Solid Edge part; units mm, degrees
sketch "Sketch1" plane through (0, 0, 0) normal (1, 0, 0) x (0, 1, 0)
  line L0 (27.5, -27) -> (27.5, 23)
  line L1 (27.5, 23) -> (-31.5, 23)
  line L2 (-31.5, 23) -> (-31.5, -27)
  line L3 (-31.5, -27) -> (27.5, -27)
extrude "Protrusion1" add sketch "Sketch1" along normal blind 2
sketch "Sketch2" plane through (0, 0, 0) normal (1, 0, 0) x (0, 1, 0)
  line L0 (-31.5, 21) -> (-7, 21)
  line L1 (-7, 21) -> (-7, 23)
  line L2 (-7, 23) -> (-31.5, 23)
  line L3 (-31.5, 23) -> (-31.5, 21)
extrude "ExtrudedCutout_1" cut sketch "Sketch2" along normal blind 2
sketch "Sketch3" plane through (0, 0, 0) normal (1, 0, 0) x (0, 1, 0)
  line L0 (3, 21) -> (27.5, 21)
  line L1 (27.5, 21) -> (27.5, 23)
  line L2 (27.5, 23) -> (3, 23)
  line L3 (3, 23) -> (3, 21)
extrude "ExtrudedCutout_2" cut sketch "Sketch3" along normal blind 2
sketch "Sketch4" plane through (0, 0, 0) normal (1, 0, 0) x (0, 1, 0)
  line L0 (23.5, 3) -> (23.5, -7)
  line L1 (23.5, -7) -> (25.5, -7)
  line L2 (25.5, -7) -> (25.5, 3)
  line L3 (25.5, 3) -> (23.5, 3)
extrude "ExtrudedCutout_3" cut sketch "Sketch4" along normal blind 2
sketch "Sketch5" plane through (0, 0, 0) normal (1, 0, 0) x (0, 1, 0)
  line L0 (27.5, -25) -> (3, -25)
  line L1 (3, -25) -> (3, -27)
  line L2 (3, -27) -> (27.5, -27)
  line L3 (27.5, -27) -> (27.5, -25)
extrude "ExtrudedCutout_4" cut sketch "Sketch5" along normal blind 4
sketch "Sketch6" plane through (0, 0, 0) normal (1, 0, 0) x (0, 1, 0)
  line L0 (-7, -25) -> (-31.5, -25)
  line L1 (-31.5, -25) -> (-31.5, -27)
  line L2 (-31.5, -27) -> (-7, -27)
  line L3 (-7, -27) -> (-7, -25)
extrude "ExtrudedCutout_5" cut sketch "Sketch6" along normal blind 2
sketch "Sketch7" plane through (0, 0, 0) normal (1, 0, 0) x (0, 1, 0)
  line L0 (-29.5, -7) -> (-27.5, -7)
  line L1 (-27.5, -7) -> (-27.5, 3)
  line L2 (-27.5, 3) -> (-29.5, 3)
  line L3 (-29.5, 3) -> (-29.5, -7)
extrude "ExtrudedCutout_6" cut sketch "Sketch7" along normal blind 4
sketch "Sketch8" plane through (0, 0, 0) normal (1, 0, 0) x (0, 1, 0)
  line L0 (7.25, 9) -> (-11.25, 9)
  line L1 (-11.25, 9) -> (-11.25, -1)
  line L2 (-11.25, -1) -> (7.25, -1)
  line L3 (7.25, -1) -> (7.25, 9)
  circle A0 centre (-14.495, 4) radius 1.98
  circle A1 centre (10.495, 4) radius 1.98
extrude "ExtrudedCutout_9" cut sketch "Sketch8" along normal blind 2
properties material "Acrylic, high impact grade"
Here's how the part is built. I have some questions about the finished solid (model axes, mm). A direction names the side the tool comes from. Give positions to 0.01 mm unless a question says otherwise; leave off trailing zeros. Write each loop counter-clockwise with the first axis right and the second up, starting at its lowest first coordinate (ties: lowest second). Pieces come first, ordered by that corner, then holes. Notation, with made-up numbers: (43.5, -18) -> (49.5, -18) arc R13 cw to (49.5, 4) -> close; hole circle Ø5 at (42, -20.75). An arc over 180 degrees is marked (long way). Use one line per item in the form item = value. Start each with the question number.
1. Imagine slicing it at A-A on z = 4. List the corners of the cut face in (x, y) for me (3 decimals).
2. If I drill on L1, parallel to Y at x = 1.1, z = -0.5; L2, parallel to Z at x = 1.35, y = 0; L3, parallel to Z at x = 1.3, y = 18.5, over which ranges is the centre line in solid material (lowest first)?
3. Imagine slicing it at D-D on y = 13.5. List the corners of the cut face in (x, z) for me.
4. Imagine slicing it at C-C on x = 1.6. List the corners of the cut face in (y, z) for me (3 decimals).
5. Thinking about a two-plate mould opening in Z: for faces 4 (the face through (0.99, -15.95, 2.66)), 5 (the face through (1, -2, -27)), 6 (the face through (1, -7, 22)), which applies, +Z half, -Z half, draft (parallel to the pull), parting line (faces both ways), or undercut?
6. Imagine slicing it at B-B on z = -6. List the corners of the cut face in (x, y) for me, plus the area to 3 significant figures.
7. Will these pins go through, and if not, where does the flat tip stop? pin 1 Ø1 at (x, y) = (1.5, 24) entering from +Z; pin 2 Ø1 at (x, y) = (0.5, 17.5) entering from -Z; pin 3 Ø1.5 at (y, z) = (-11.5, 0.5) entering from -X; pin 4 Ø0.6 at (x, z) = (1, -26) entering from -Y.
8. On a 3-axis mill with a long thin cutter (end or side, diameter ignored), from which of +Z, -Z, +X, -X, +Y, -Y can I reach the whole of each face in a straight line? I mean faces 1 (the face through (1, 15, -25)), 2 (the face through (1, -2, 9)), 3 (the face through (1, -19, 21)). Say none if no direction works.
Entries:
q1.outline = (0, -31.5) -> (2, -31.5) -> (2, -16.475) -> (0, -16.475) -> close; (0, -12.515) -> (2, -12.515) -> (2, -11.25) -> (0, -11.25) -> close; (0, 7.25) -> (2, 7.25) -> (2, 8.515) -> (0, 8.515) -> close; (0, 12.475) -> (2, 12.475) -> (2, 27.5) -> (0, 27.5) -> close
q2.L1 = -31.5 to -29.5, -27.5 to -11.25, 7.25 to 23.5, 25.5 to 27.5
q2.L2 = -27 to -1, 9 to 23
q2.L3 = -25 to 21
q3.outline = (0, -25) -> (2, -25) -> (2, 21) -> (0, 21) -> close
q4.outline = (-31.5, -25) -> (-7, -25) -> (-7, -27) -> (3, -27) -> (3, -25) -> (27.5, -25) -> (27.5, 21) -> (3, 21) -> (3, 23) -> (-7, 23) -> (-7, 21) -> (-31.5, 21) -> close; hole (-29.5, -7) -> (-27.5, -7) -> (-27.5, 3) -> (-29.5, 3) -> close; hole circle Ø3.96 at (-14.495, 4); hole (-11.25, -1) -> (7.25, -1) -> (7.25, 9) -> (-11.25, 9) -> close; hole circle Ø3.96 at (10.495, 4); hole (23.5, -7) -> (25.5, -7) -> (25.5, 3) -> (23.5, 3) -> close
q5.face_4 = undercut
q5.face_5 = -Z half
q5.face_6 = draft
q6.outline = (0, -31.5) -> (2, -31.5) -> (2, -29.5) -> (0, -29.5) -> close; (0, -27.5) -> (2, -27.5) -> (2, 23.5) -> (0, 23.5) -> close; (0, 25.5) -> (2, 25.5) -> (2, 27.5) -> (0, 27.5) -> close
q6.area = 110 mm²
q7.pin_1 = 21
q7.pin_2 = -25
q7.pin_3 = 0
q7.pin_4 = -7
q8.face_1 = -Z, +X, -X, +Y
q8.face_2 = +X, -X
q8.face_3 = +Z, +X, -X, -Y
